Build history of the part. All positions in model axes, mm. Face numbers are marked on the shaded views. Give positions to 0.01 mm unless a question says otherwise; leave off trailing zeros. Loops run counter-clockwise (first coordinate to the right, second up) from the corner with the lowest first, then second, coordinate; pieces in that order, holes last. Notation, with made-up numbers: M 32.25,-36 L 69.25,-36 A22 ccw 69.25,-8 Z; hole C 55,14 d2. An arc over 180 degrees is marked long. Put each result on its own line as item: value.
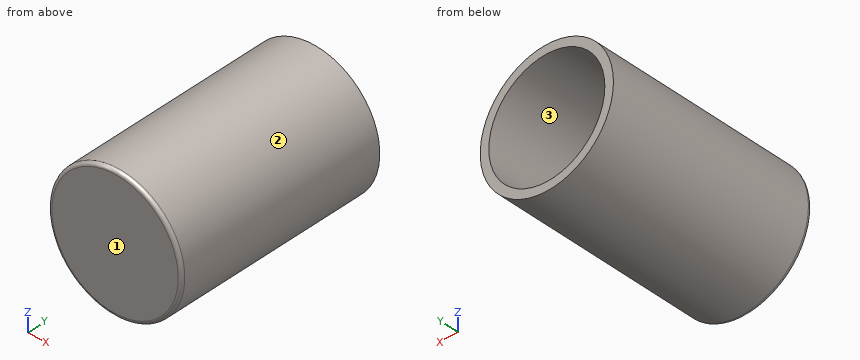
Autodesk Inventor part; units mm, degrees
ref_plane "YZ Plane" through (0, 0, 0) normal (1, 0, 0) x (0, 1, 0)
ref_plane "XZ Plane" through (0, 0, 0) normal (0, 1, 0) x (-1, 0, 0)
ref_plane "XY Plane" through (0, 0, 0) normal (0, 0, 1) x (1, 0, 0)
sketch "Sketch1" plane through (0, 0, 0) normal (0, 1, 0) x (-1, 0, 0)
  circle A0 centre (0, 0) radius 38.75
  dimension "d0" = 77.5
extrude "Extrusion1" add sketch "Sketch1" along normal blind 125
shell "Shell1" thickness 5 removed faces 1 at (-4.4693, 125, 5.6043)
fillet "Fillet1" radius 2 2 edges at (33.75, 5, 0) (38.75, 0, 0)
properties part number "Inner Layer"
Q1. Mould opens along Z. For the marked faces 1, 2 and 3 say: pulls with the +Z half, pulls with the -Z half, needs draft (parallel to the pull), parting line crosses it, or undercut.
Here are the results:
face 1: needs draft
face 2: parting line crosses it
face 3: undercut
Q2. Slice it at A-A (z = 0). List the corners of the cut face in (x, y).
Here are the results:
outline: M -38.75,2 A2 ccw -36.75,0 L 36.75,0 A2 ccw 38.75,2 L 38.75,125 L 33.75,125 L 33.75,7 A2 cw 31.75,5 L -31.75,5 A2 cw -33.75,7 L -33.75,125 L -38.75,125 Z
Q3. Probe line 1 (Z direction, x = 1, y = 104); line 2 (X direction, y = 86, z = 0.5); line 3 (Y direction, x = -15, z = 19). List the from-to ranges inside material, lowest first. Write a range as from..to.
Here are the results:
line 1: -38.74..-33.74, 33.74..38.74
line 2: -38.75..-33.75, 33.75..38.75
line 3: 0..5
Q4. Drop flat-ended pins along their axis: pin 1 Ø6 at (x, y) = (-16, 35.5) entering from +Z; pin 2 Ø10 at (x, y) = (6.5, 39.5) entering from +Z; pin 3 Ø10 at (x, y) = (20, 75.5) entering from -Z. Give the stop position or say it passes through.
Here are the results:
pin 1: z = 36.5
pin 2: z = 38.72
pin 3: z = -35.73
Q5. Slice it at C-C (y = 26). List the corners of the cut face in (x, z), and give its area (3 significant figures).
Here are the results:
outline: C 0,0 d77.5; hole C 0,0 d67.5
area: 1,140 mm²
Q6. Slice it at B-B (x = 0). List the corners of the cut face in (y, z).
Here are the results:
outline: M 0,-36.75 A2 ccw 2,-38.75 L 125,-38.75 L 125,-33.75 L 7,-33.75 A2 cw 5,-31.75 L 5,31.75 A2 cw 7,33.75 L 125,33.75 L 125,38.75 L 2,38.75 A2 ccw 0,36.75 Z
